Design review of the part built by this model. Coordinates are the model's own, in mm. A direction names the side the tool comes from. Give positions to 0.01 mm unless a question says otherwise; leave off trailing zeros. Loops run counter-clockwise (first coordinate to the right, second up) from the corner with the lowest first, then second, coordinate; pieces in that order, holes last. Notation, with made-up numbers: M 15,-28 L 66,-28 A7 cw 66,-21 Z; hole C 88,64 d9. An arc over 180 degrees is marked long. Use CSV: the item, a comma, the result in double quotes.
from build123d import *

# Parameters (mm, degrees)
SKETCH_W        = 30
SKETCH_H        = 26
PAD_DEPTH       = 6
SKETCH001_W     = 46
SKETCH001_H     = 21
POCKET_DEPTH    = 3.5
SKETCH003_W     = 20
SKETCH003_H     = 20
PAD001_DEPTH    = 18.5
SKETCH004_R     = 6.2
POCKET001_DEPTH = 14
POCKET002_DEPTH = 3.5
SKETCH006_R     = 2.5
POCKET003_DEPTH = 6.001
FILLET_R        = 5


with BuildPart() as part:
    # Sketch → Pad (new body)
    with BuildSketch(Plane.XY):
        Rectangle(SKETCH_W, SKETCH_H)
    extrude(amount=PAD_DEPTH)

    # Sketch001 (on Face5 of Pad) → Pocket (cut)
    with BuildSketch(Plane(origin=(0, 0, 0), x_dir=(1, 0, 0), z_dir=(0, 0, -1))):
        Rectangle(SKETCH001_W, SKETCH001_H)
    extrude(amount=-POCKET_DEPTH, mode=Mode.SUBTRACT)

    # Sketch003 → Pad001 (join)
    with BuildSketch(Plane.XY.offset(5)):
        Rectangle(SKETCH003_W, SKETCH003_H)
    extrude(amount=PAD001_DEPTH)

    # Sketch004 (on Face15 of Pad001) → Pocket001 (cut)
    with BuildSketch(Plane.XY.offset(23.5)):
        Circle(SKETCH004_R)
    extrude(amount=-POCKET001_DEPTH, mode=Mode.SUBTRACT)

    # Sketch005 (on Face17 of Pocket001) → Pocket002 (cut)
    with BuildSketch(Plane.XY.offset(9.5)):
        Polygon((2.107328, -3.65), (4.214657, 0), (2.107328, 3.65), (-2.107328, 3.65), (-4.214657, 0), (-2.107328, -3.65), align=None)
    extrude(amount=-POCKET002_DEPTH, mode=Mode.SUBTRACT)

    # Sketch006 (on Face24 of Pocket002) → Pocket003 (cut, through all)
    with BuildSketch(Plane.XY.offset(6)):
        Circle(SKETCH006_R)
    extrude(amount=-POCKET003_DEPTH, mode=Mode.SUBTRACT)

    # Fillet
    fillet_edges = [part.edges().sort_by_distance(p)[0] for p in [
        (-10, 10, 14.75),
        (10, 10, 14.75),
        (10, -10, 14.75),
        (-10, -10, 14.75),
    ]]
    fillet(fillet_edges, radius=FILLET_R)


solid = part.part
(1) We need section D-D on x = -12.5. State the section outline as (y, z) points, then the cut area to 3 significant figures.
A:
outline,"M -13,0 L -10.5,0 L -10.5,3.5 L 10.5,3.5 L 10.5,0 L 13,0 L 13,6 L -13,6 Z"
area,"82.5 mm²"
(2) We need section A-A on x = 0. State the section outline as (y, z) points.
A:
outline,"M -13,0 L -10.5,0 L -10.5,3.5 L -2.5,3.5 L -2.5,6 L -3.65,6 L -3.65,9.5 L -6.2,9.5 L -6.2,23.5 L -10,23.5 L -10,6 L -13,6 Z; M 2.5,3.5 L 10.5,3.5 L 10.5,0 L 13,0 L 13,6 L 10,6 L 10,23.5 L 6.2,23.5 L 6.2,9.5 L 3.65,9.5 L 3.65,6 L 2.5,6 Z"
(3) We need section C-C on y = -8. State the section outline as (x, z) points, then the cut area to 3 significant figures.
A:
outline,"M -15,3.5 L 15,3.5 L 15,6 L 9,6 L 9,23.5 L -9,23.5 L -9,6 L -15,6 Z"
area,"390 mm²"
(4) The part is to be moulded in two halves that separate along Y. For faces 1 (the flat face through (0, 13, 3)), 2 (the flat face through (0, -10, 15)), 3 (the flat face through (0, 3.65, 8)), say which applies: released by +Y, released by -Y, zero draft, split by the parting line, or undercut.
A:
face 1,"released by +Y"
face 2,"released by -Y"
face 3,"undercut"
(5) We need section B-B on z = 17.75. State the section outline as (x, y) points, then the cut area to 3 significant figures.
A:
outline,"M -10,-5 A5 ccw -5,-10 L 5,-10 A5 ccw 10,-5 L 10,5 A5 ccw 5,10 L -5,10 A5 ccw -10,5 Z; hole C 0,0 d12.4"
area,"258 mm²"
(6) Clearance check with flat-ended pins moving along their axes: P1, Ø1.5, axis at x = 9.5, y = 9, coming from the -Z side; P2, Ø3, axis at y = 1.5, z = 13, coming from the -X side; P3, Ø5, axis at x = -2, z = 9.5, coming from the -Y side. State where each tip first meets the part, or that it passes through.
A:
P1,"z = 3.5"
P2,"x = -10"
P3,"y = -10"
(7) Machinability: for faces 4 (the flat face through (-10, 0, 15)), 5 (the flat face through (0, -3.65, 8)), 6 (the flat face through (10, 0, 15)), 7 (the cylindrical face through (8, 9, 15)), which of the approach directions +Z, -Z, +X, -X, +Y, -Y give a long, thin tool a straight path to every point of the face, cutting with its end or side? Answer none if there is none.
A:
face 4,"+Z, -X, +Y, -Y"
face 5,"+Z"
face 6,"+Z, +X, +Y, -Y"
face 7,"+Z, +X, +Y"
(8) Wall thickness on line 1 along Y through (x, z) = (0, 4.5); line 2 along Y through (x, z) = (-1.5, 6.75); line 3 along Z through (x, y) = (1.25, 9.25): over which ranges is each line inside the solid? List them lowest first. Write a range as [from, to].
A:
line 1,"[-13, -2.5], [2.5, 13]"
line 2,"[-10, -3.65], [3.65, 10]"
line 3,"[3.5, 23.5]"
